Autodesk Inventor part; units mm, degrees
ref_plane "YZ Plane" through (0, 0, 0) normal (1, 0, 0) x (0, 1, 0)
ref_plane "XZ Plane" through (0, 0, 0) normal (0, 1, 0) x (-1, 0, 0)
ref_plane "XY Plane" through (0, 0, 0) normal (0, 0, 1) x (1, 0, 0)
sketch "Sketch1" plane through (0, 0, 0) normal (0, 0, 1) x (1, 0, 0)
  circle A0 centre (0, 0) radius 28
  circle A1 centre (0, 0) radius 1.8
  arc A2 (23.4652, 15.2769) -> (5.1796, 27.5168) centre (0, 0) ccw
  arc A3 (1.1742, 1.3642) -> (0.0115, 1.8) centre (0, 0) ccw
  arc A4 (1.3642, -1.1742) -> (1.8, -0.0115) centre (0, 0) ccw
  arc A5 (-1.3642, 1.1742) -> (-1.8, 0.0115) centre (0, 0) ccw
  arc A6 (-1.1742, -1.3642) -> (-0.0115, -1.8) centre (0, 0) ccw
  arc A7 (8.0598, 19.9487) -> (-0.0006, 1.8) centre (26.4682, 0.9087) ccw
  arc A8 (23.1644, 13.6701) -> (13.3624, 21.0083) centre (4.9305, -0.4702) ccw
  arc A9 (19.6092, 5.6217) -> (1.6116, 0.8017) centre (23.6763, -45.5755) ccw
  arc A10 (1.6116, 0.8017) -> (-0.0006, 1.8) centre (0, 0) ccw
  arc A11 (13.3624, 21.0083) -> (8.0598, 19.9487) centre (11.5352, 16.3541) ccw
  arc A12 (19.6092, 5.6217) -> (23.1644, 13.6701) centre (19.2133, 10.606) ccw
  arc A13 (19.9487, -8.0598) -> (1.8, 0.0006) centre (0.9087, -26.4682) ccw
  arc A14 (13.6701, -23.1644) -> (21.0083, -13.3624) centre (-0.4702, -4.9305) ccw
  arc A15 (5.6217, -19.6092) -> (0.8017, -1.6116) centre (-45.5755, -23.6763) ccw
  arc A16 (0.8017, -1.6116) -> (1.8, 0.0006) centre (0, 0) ccw
  arc A17 (21.0083, -13.3624) -> (19.9487, -8.0598) centre (16.3541, -11.5352) ccw
  arc A18 (5.6217, -19.6092) -> (13.6701, -23.1644) centre (10.606, -19.2133) ccw
  arc A19 (-1.1742, -1.3642) -> (-0.0115, -1.8) centre (0, 0) ccw
  arc A20 (-8.0598, -19.9487) -> (0.0006, -1.8) centre (-26.4682, -0.9087) ccw
  arc A21 (-23.1644, -13.6701) -> (-13.3624, -21.0083) centre (-4.9305, 0.4702) ccw
  arc A22 (-19.6092, -5.6217) -> (-23.1644, -13.6701) centre (-19.2133, -10.606) ccw
  arc A23 (-13.3624, -21.0083) -> (-8.0598, -19.9487) centre (-11.5352, -16.3541) ccw
  arc A24 (-19.6092, -5.6217) -> (-1.6116, -0.8017) centre (-23.6763, 45.5755) ccw
  arc A25 (-1.6116, -0.8017) -> (0.0006, -1.8) centre (0, 0) ccw
  arc A26 (-19.9487, 8.0598) -> (-1.8, -0.0006) centre (-0.9087, 26.4682) ccw
  arc A27 (-21.0083, 13.3624) -> (-19.9487, 8.0598) centre (-16.3541, 11.5352) ccw
  arc A28 (-5.6217, 19.6092) -> (-0.8017, 1.6116) centre (45.5755, 23.6763) ccw
  arc A29 (-13.6701, 23.1644) -> (-21.0083, 13.3624) centre (0.4702, 4.9305) ccw
  arc A30 (-5.6217, 19.6092) -> (-13.6701, 23.1644) centre (-10.606, 19.2133) ccw
  arc A31 (-0.8017, 1.6116) -> (-1.8, -0.0006) centre (0, 0) ccw
  circle A32 centre (0, 0) radius 1
  point P0 (0.0006, -1.8)
  point P1 (-1.6116, -0.8017)
  point P2 (-1.8, -0.0006)
  point P3 (-0.8017, 1.6116)
  point P4 (1.8, 0.0006)
  point P5 (0.8017, -1.6116)
  dimension "d2" = 5
  dimension "d3" = 5
  dimension "d4" = 5
  dimension "d5" = 5
  dimension "d6" = 5
  dimension "d7" = 5
  dimension "d8" = 5
  dimension "d9" = 5
  dimension "d15" = 3.6
  dimension "d16" = 2
extrude "Extrusion1" add sketch "Sketch1" along normal blind 1 contours A13 A17 A14 A18 A15 A1 | A1 A7 A11 A8 A12 A9 | A20 A23 A21 A22 A24 A1 | A1 A26 A27 A29 A30 A28
sketch "Sketch2" plane through (0, 0, 0) normal (1, 0, 0) x (0, 1, 0)
  line L0 (0.9994, 0) -> (2.7994, 0)
  line L1 (2.7994, 0) -> (2.7994, 1)
  line L2 (2.7994, 1) -> (0.9994, 1)
  line L3 (0.9994, 1) -> (0.9994, 0)
  line L4 (0, -0.2) -> (0, 1.2)
  point P0 (0, 0)
  dimension "d12" = 1.8
  dimension "d13" = 1
revolve "Revolution1" add sketch "Sketch2" angle 360 about axis through (0, 0, -10) along (0, 0, 1)
properties part number "blades"
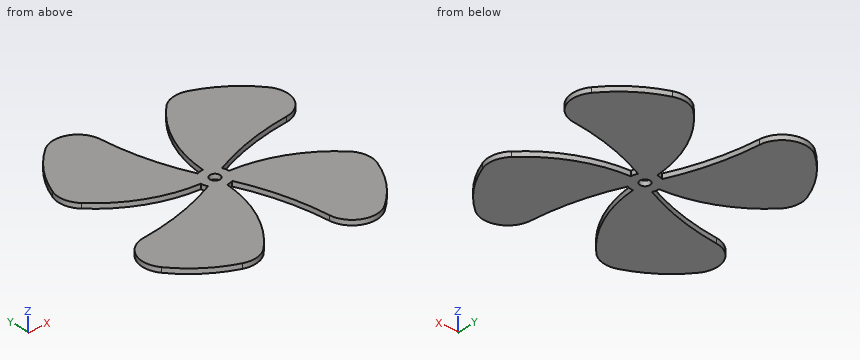
Verification items for the finished model (mm, model axes). Give positions to 0.01 mm unless a question says otherwise; leave off trailing zeros. Order: outer loops, then holes, each group sorted by start corner. A loop starts at its lowest first (then second) coordinate and runs counter-clockwise, first axis right, second up. Notation, with made-up numbers: M 59.25,69.5 L 110.25,69.5 A15 ccw 110.25,74.5 Z; hole C 32,21.5 d7. An arc over 180 degrees is marked long. Use one line per item in the form item = value. Start each with the question number.
Q1. Scan lines: line 1 along X through (y, z) = (0, 0.35); line 2 along Y through (x, z) = (17, 0.55). Record each from-to range of solid material in increasing order. Write a range as [from, to].
Q2. Section check B-B (x = 12). Enter the section's corners in (y, z), then the cut area to 3 significant figures.
Q3. Section check A-A (z = 0.6). Enter the section's corners in (x, y), then the cut area to 3 significant figures.
Q4. Section check C-C (y = -4). Enter the section's corners in (x, z), then the cut area to 3 significant figures.
Evaluation:
q1.line_1 = [-2.8, -1], [1, 2.8]
q1.line_2 = [-20, -5.43], [5.35, 19.2]
q2.outline = M -24.02,0 L -2.42,0 L -2.42,1 L -24.02,1 Z; M 4.44,0 L 21.33,0 L 21.33,1 L 4.44,1 Z
q2.area = 38.5 mm2
q3.outline = M -23.16,-13.67 A23.07 ccw -13.36,-21.01 A5 ccw -8.06,-19.95 A26.48 ccw -0.05,-2.8 A2.8 ccw 1.22,-2.52 A51.36 cw 5.62,-19.61 A5 ccw 13.67,-23.16 A23.07 ccw 21.01,-13.36 A5 ccw 19.95,-8.06 A26.48 ccw 2.8,-0.05 A2.8 ccw 2.52,1.22 A51.36 cw 19.61,5.62 A5 ccw 23.16,13.67 A23.07 ccw 13.36,21.01 A5 ccw 8.06,19.95 A26.48 ccw 0.05,2.8 A2.8 ccw -1.22,2.52 A51.36 cw -5.62,19.61 A5 ccw -13.67,23.16 A23.07 ccw -21.01,13.36 A5 ccw -19.95,8.06 A26.48 ccw -2.8,0.05 A2.8 ccw -2.52,-1.22 A51.36 cw -19.61,-5.62 A5 ccw Z; hole C 0,0 d2
q3.area = 1,260 mm2
q4.outline = M -10.26,0 L -0.17,0 L -0.17,1 L -10.26,1 Z; M 1.86,0 L 14.93,0 L 14.93,1 L 1.86,1 Z
q4.area = 23.2 mm2
